Here's how the part is built. I have some questions about the finished solid (model axes, mm). Give positions to 0.01 mm unless a question says otherwise; leave off trailing zeros. Loops run counter-clockwise (first coordinate to the right, second up) from the corner with the lowest first, then second, coordinate; pieces in that order, holes last. Notation, with made-up numbers: (-39, -24.5) - (-8, -24.5) arc R29 cw to (-8, 9.5) - close; hole circle Ø11 at (-27, 30.25). An arc over 180 degrees is marked (long way). Use a Markdown table: item, result.
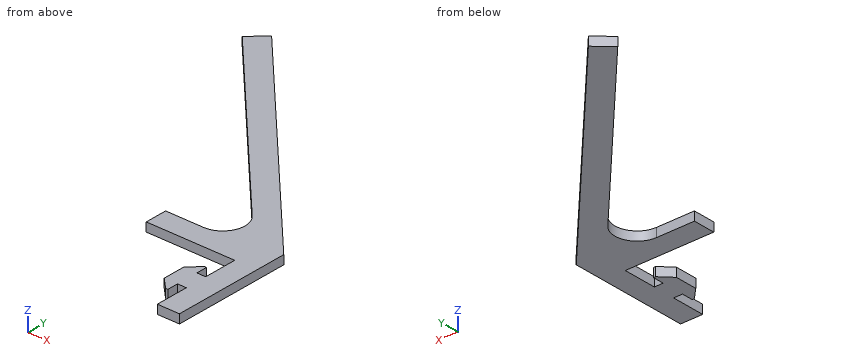
from build123d import *

# Parameters (mm, degrees)
F1_DEPTH = 2
F2_R     = 5


with BuildPart() as f1:
    # F0 (on Top) → F1 (new body)
    with BuildSketch(Plane.XY):
        Polygon((-27.900762, 36.815232), (-27.900762, 31.815232), (-7.900762, 31.815232), (-7.900762, 24.315232), (-9.900762, 24.315232), (-9.900762, 26.815232), (-10.400762, 26.815232), (-12.900762, 24.315232), (-12.900762, 19.315232), (-10.400762, 16.815232), (-9.900762, 16.815232), (-9.900762, 19.315232), (-7.900762, 19.315232), (-7.900762, 11.815232), (-2.900762, 11.815232), (-2.900762, 38.772724), (-53.820934, 93.837559), (-57.491923, 90.442881), (-7.900762, 36.815232), align=None)
    extrude(amount=F1_DEPTH)

    # F2
    f2_edges = [f1.edges().sort_by_distance(p)[0] for p in [
        (-7.900762, 36.815232, 1),
    ]]
    fillet(f2_edges, radius=F2_R)


solid = f1.part
(1) Will these pins go through, and if not, where does the flat tip stop? pin 1 (1 mm diameter, centred on x = -22.5, z = 0.5, fed in from +Y); pin 2 (1 mm diameter, centred on y = 22.5, z = 1, fed in from -X); pin 3 (1 mm diameter, centred on y = 27.5, z = 0.5, fed in from -X).
A:
| item | result |
|---|---|
| pin 1 | y = 60.51 |
| pin 2 | x = -12.9 |
| pin 3 | x = -7.9 |
(2) Suppose I cut it at D-D on y = 36. Write out the boundary of the cut face in (x, z).
A:
| item | result |
|---|---|
| outline | (-27.9, 0) - (-2.9, 0) - (-2.9, 2) - (-27.9, 2) - close |
(3) Suppose I cut it at C-C on z = 1.6. Write out the boundary of the cut face in (x, y), plus the area to 3 significant figures.
A:
| item | result |
|---|---|
| outline | (-57.49, 90.44) - (-15.66, 45.21) arc R5 cw to (-19.33, 36.82) - (-27.9, 36.82) - (-27.9, 31.82) - (-7.9, 31.82) - (-7.9, 24.32) - (-9.9, 24.32) - (-9.9, 26.82) - (-10.4, 26.82) - (-12.9, 24.32) - (-12.9, 19.32) - (-10.4, 16.82) - (-9.9, 16.82) - (-9.9, 19.32) - (-7.9, 19.32) - (-7.9, 11.82) - (-2.9, 11.82) - (-2.9, 38.77) - (-53.82, 93.84) - close |
| area | 662 mm2 |
(4) Suppose I cut it at B-B on x = -11.5. Write out the boundary of the cut face in (y, z), plus the area to 3 significant figures.
A:
| item | result |
|---|---|
| outline | (17.91, 0) - (25.72, 0) - (25.72, 2) - (17.91, 2) - close; (31.82, 0) - (48.07, 0) - (48.07, 2) - (31.82, 2) - close |
| area | 48.1 mm2 |
(5) Suppose I cut it at A-A on y = 18. Write out the boundary of the cut face in (x, z), plus the area to 3 significant figures.
A:
| item | result |
|---|---|
| outline | (-11.59, 0) - (-9.9, 0) - (-9.9, 2) - (-11.59, 2) - close; (-7.9, 0) - (-2.9, 0) - (-2.9, 2) - (-7.9, 2) - close |
| area | 13.4 mm2 |
(6) If I drill on line 1 (Y direction, x = -11, z = 1.85); line 2 (Y direction, x = -25.5, z = 1.8); line 3 (X direction, y = 61, z = 1.05), over which ranges is the centre line in solid material (lowest first)?
A:
| item | result |
|---|---|
| line 1 | 17.41 to 26.22, 31.82 to 47.53 |
| line 2 | 31.82 to 36.82, 55.85 to 63.21 |
| line 3 | -30.27 to -23.46 |
